from build123d import *

# Parameters (mm, degrees)
F0_W     = 63.5
F0_H     = 63.5
F1_DEPTH = 63.5
F2_W     = 45.72
F2_H     = 45.72
F3_DEPTH = 44.76763
F4_R     = 7.62


with BuildPart() as f1:
    # F0 (on Front) → F1 (new body)
    with BuildSketch(Plane.XZ):
        Rectangle(F0_W, F0_H)
    extrude(amount=F1_DEPTH)

    # F2 (on face) → F3 (cut)
    with BuildSketch(Plane.XZ.offset(63.5)):
        with Locations((8.89, -8.89)):
            Rectangle(F2_W, F2_H)
    extrude(amount=-F3_DEPTH, mode=Mode.SUBTRACT)

    # F4
    f4_edges = [f1.edges().sort_by_distance(p)[0] for p in [
        (-31.75, 0, 0),
        (-31.75, -31.75, 31.75),
        (0, 0, 31.75),
    ]]
    fillet(f4_edges, radius=F4_R)


solid = f1.part
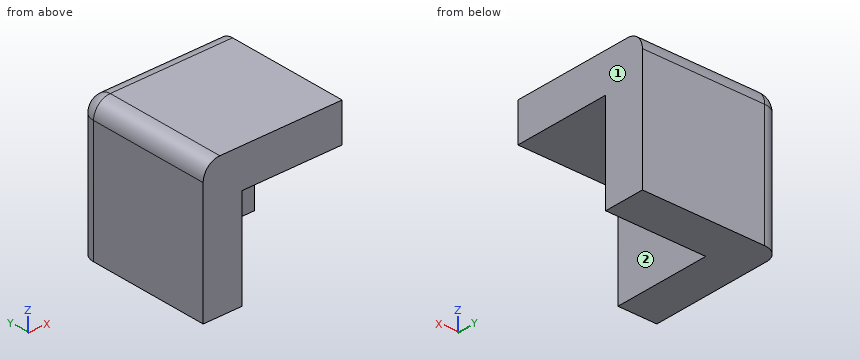
Input: part model. Units: mm. Frame: model coordinates. Face numbers are marked on the shaded views. A direction names the side the tool comes from. Round coordinates to 2 decimals unless told otherwise and drop trailing zeros. Order: outer loops, then holes, each group sorted by start corner. A loop starts at its lowest first (then second) coordinate and runs counter-clockwise, first axis right, second up. Notation, with made-up numbers: (14.5, 41.25) - (26.5, 41.25) arc R29 ccw to (26.5, 63.25) - close; hole circle Ø3 at (70, 15). An arc over 180 degrees is marked (long way). Answer as a JSON object with one key per item and string values. Group by question number.
(1) Material intervals for probe 1 along X at (y, z) = (-28, 9.5); probe 2 along Y at (x, z) = (-12, 10); probe 3 along Z at (x, y) = (-24.5, -57), sorted ascending. Write a range as from..to.
(2) Cut plane C-C (y = -4). Return loops of the section in (x, z).
(3) Pin query (flat end, axial travel): P1, Ø2, axis at y = -57, z = -16.5, coming from the +X side; P2, Ø12, axis at x = -7.5, z = -4, coming from the -Y side; P3, Ø8, axis at x = 12, y = -54.5, coming from the -Z side. Return the tip coordinate at first contact, or that it passes through.
(4) Cut plane B-B (y = -58.5). Return loops of the section in (x, z).
(5) Cut plane A-A (z = 3). Return loops of the section in (x, y), then the cut area to 3 significant figures.
(6) Reachability of the marked faces 1 and 2 from +Z, -Z, +X, -X, +Y, -Y: full face, straight path, thin tool, end or side. Return the list, or none.
Here are the results:
{
 "1": {"probe 1": "x = -31.75..-13.97", "probe 2": "y = -18.73..0", "probe 3": "z = -31.75..31.74"},
 "2": {"outline": "(-30.84, -31.75) - (31.75, -31.75) - (31.75, 30.84) - (-24.13, 30.84) arc R6.71 ccw to (-30.84, 24.13) - close"},
 "3": {"P1": "stops at x = -13.97", "P2": "stops at y = -18.73", "P3": "stops at z = 13.97"},
 "4": {"outline": "(-31.75, -31.75) - (-13.97, -31.75) - (-13.97, 13.97) - (31.75, 13.97) - (31.75, 31.75) - (-24.13, 31.75) arc R7.62 ccw to (-31.75, 24.13) - close"},
 "5": {"outline": "(-31.75, -63.5) - (-13.97, -63.5) - (-13.97, -18.73) - (31.75, -18.73) - (31.75, 0) - (-24.13, 0) arc R7.62 ccw to (-31.75, -7.62) - close", "area": "1,970 mm^2"},
 "6": {"face 1": "+Z, -Z, +X, +Y, -Y", "face 2": "-Z, +X, -Y"}
}
